Job drawing, mm, ordinate dimensions from the low corner. One solid piece. A direction names the side the tool comes from. Give positions to 0.01 mm unless a question says otherwise; leave off trailing zeros. Order: outer loops, then holes, each group sorted by start corner. A loop starts at its lowest first (then second) coordinate and runs counter-clockwise, first axis right, second up.
1. Drop flat-ended pins along their axis: pin 1 Ø6 at (y, z) = (3, 6.5) entering from +X; pin 2 Ø6 at (x, z) = (3, 10.5) entering from -Y; pin 3 Ø2 at (x, z) = (7, 3) entering from +Y; pin 4 Ø1 at (y, z) = (9, 10) entering from +X. Give the stop position or say it passes through.
2. Slice it at A-A on y = 3.75. List the corners of the cut face in (x, z).
3. Mould opens along X. For the marked faces 3, 4 and 5 say: +X half, -X half, draft (parallel to the pull), parting line (faces both ways), or undercut.
4. Probe line 1 (X direction, y = 9.5, z = 6.5); line 2 (Y direction, x = 10.75, z = 2.75) (1 decimal); line 3 (Y direction, x = 4, z = 9.5). List the from-to ranges inside material, lowest first.
5. Which spindle directions (+Z, -Z, +X, -X, +Y, -Y) get a long thin tool onto all of the face, cutting with end or side? Do the marked faces 1 and 2. Say none if no direction does.
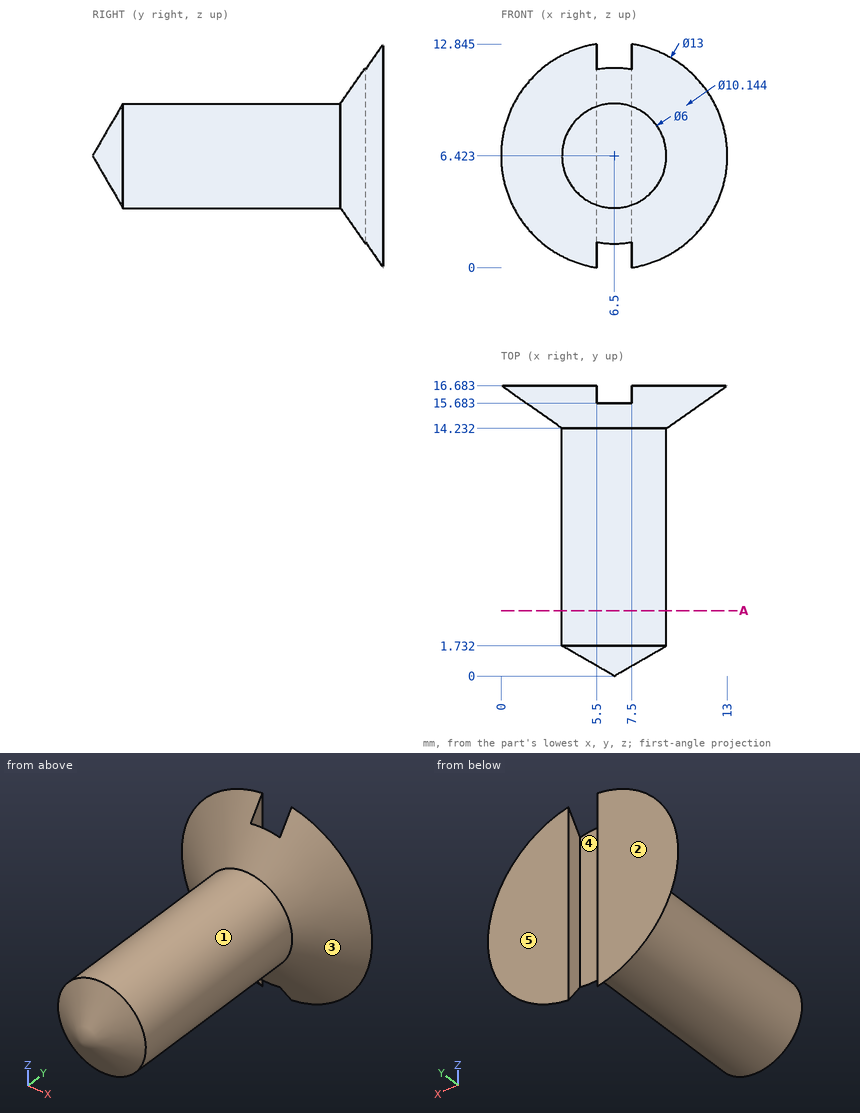
Data:
1. pin 1: stops at x = 9.5
1. pin 2: stops at y = 1.37
1. pin 3: stops at y = 16.68
1. pin 4: passes through
2. outline: circle Ø6 at (6.5, 6.42)
3. face 3: parting line
3. face 4: undercut
3. face 5: draft
4. line 1: x = 3.5 to 9.5
4. line 2: y = 16.1 to 16.7
4. line 3: y = 14.91 to 16.68
5. face 1: -Y
5. face 2: +Z, -Z, +X, -X, +Y
